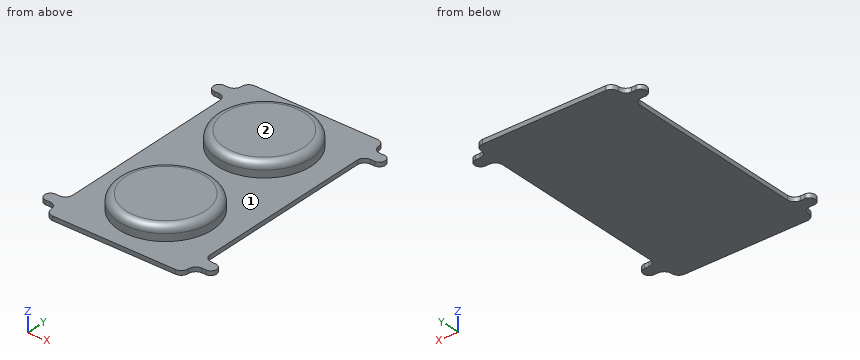
```python
from build123d import *

# Parameters (mm, degrees)
EXTRUDE_1_DEPTH = 3
FILLET_1_R      = 5
SKETCH_2_R      = 32.5
EXTRUDE_2_DEPTH = 10
FILLET_2_R      = 5


with BuildPart() as part:
    # 草圖1 → 填料-伸長1 (new body)
    with BuildSketch(Plane.XY):
        with BuildLine():
            Line((-47.5, 67), (-47.5, -67))
            Line((-47.5, -67), (-55.5, -67))
            ThreePointArc((-55.5, -67), (-59.5, -71), (-55.5, -75))
            Line((-55.5, -75), (-47.5, -75))
            Line((-47.5, -75), (-47.5, -85))
            Line((-47.5, -85), (47.5, -85))
            Line((47.5, -85), (47.5, -75))
            Line((47.5, -75), (55.5, -75))
            ThreePointArc((55.5, -75), (59.5, -71), (55.5, -67))
            Line((55.5, -67), (47.5, -67))
            Line((47.5, -67), (47.5, 67))
            Line((47.5, 67), (55.5, 67))
            ThreePointArc((55.5, 67), (59.5, 71), (55.5, 75))
            Line((55.5, 75), (47.5, 75))
            Line((47.5, 75), (47.5, 85))
            Line((47.5, 85), (-47.5, 85))
            Line((-47.5, 85), (-47.5, 75))
            Line((-47.5, 75), (-55.5, 75))
            ThreePointArc((-55.5, 75), (-59.5, 71), (-55.5, 67))
            Line((-55.5, 67), (-47.5, 67))
        make_face()
    extrude(amount=EXTRUDE_1_DEPTH)

    # 圓角1
    fillet_1_edges = [part.edges().sort_by_distance(p)[0] for p in [
        (-47.5, 85, 1.5),
        (47.5, 85, 1.5),
        (47.5, 75, 1.5),
        (47.5, 67, 1.5),
        (47.5, -67, 1.5),
        (47.5, -75, 1.5),
        (47.5, -85, 1.5),
        (-47.5, -85, 1.5),
        (-47.5, -75, 1.5),
        (-47.5, -67, 1.5),
        (-47.5, 67, 1.5),
        (-47.5, 75, 1.5),
    ]]
    fillet(fillet_1_edges, radius=FILLET_1_R - 0.0001)  # a hair under: the kernel refuses the full size

    # 草圖2 → 填料-伸長2 (add)
    with BuildSketch(Plane.XY.offset(3)):
        with Locations((0, 41.5)):
            Circle(SKETCH_2_R)
        with Locations(Location((0, -41.5, 0), (0, 0, 180))):
            Circle(SKETCH_2_R)
    extrude(amount=EXTRUDE_2_DEPTH)

    # 圓角2
    fillet_2_edges = [part.edges().sort_by_distance(p)[0] for p in [
        (-32.5, 41.5, 13),
        (32.5, -41.5, 13),
    ]]
    fillet(fillet_2_edges, radius=FILLET_2_R)


solid = part.part
```
The model under review builds one solid part; all positions refer to its coordinate system, in mm. Face numbers are marked on the shaded views. Coordinates: 2 decimals unless noted, no trailing zeros. Write each loop counter-clockwise with the first axis right and the second up, starting at its lowest first coordinate (ties: lowest second). Pieces come first, ordered by that corner, then holes.
1) The part is to be moulded in two halves that separate along Y. For the marked faces 1 and 2, say which applies: pulls with the +Y half, pulls with the -Y half, needs draft (parallel to the pull), parting line crosses it, or undercut.
2) To check wall thickness, follow probe 1 along X at (y, z) = (43, 7.25); probe 2 along Z at (x, y) = (-36.5, -24); probe 3 along Y at (x, z) = (2.5, 7.25). State the ranges of each line that lie inside material, in increasing order.
3) We need section C-C on z = 11. State the section outline as (x, y) points.
4) We need section A-A on y = -41.5. State the section outline as (x, z) points.
5) Clearance check with flat-ended pins moving along their axes: pin 1 Ø2.5 at (x, z) = (54, 1.5) entering from +Y; pin 2 Ø0.9 at (x, z) = (-53.5, 1.5) entering from -Y; pin 3 Ø1 at (x, z) = (-30, 5.5) entering from +Y. State where each tip first meets the part, or that it passes through.
6) We need section B-B on x = 0. State the section outline as (y, z) points, then the cut area to 3 significant figures.
7) We need section D-D on x = 38. State the section outline as (y, z) points.
Answer list:
1. face 1: undercut
1. face 2: needs draft
2. probe 1: x = -32.47 to 32.47
2. probe 2: z = 0 to 3
2. probe 3: y = -73.9 to -9.1, 9.1 to 73.9
3. outline: circle Ø63 at (0, -41.5); circle Ø63 at (0, 41.5)
4. outline: (-47.5, 0) - (47.5, 0) - (47.5, 3) - (32.5, 3) - (32.5, 8) arc R5 ccw to (27.5, 13) - (-27.5, 13) arc R5 ccw to (-32.5, 8) - (-32.5, 3) - (-47.5, 3) - close
5. pin 1: stops at y = 75
5. pin 2: stops at y = -75
5. pin 3: stops at y = 55.14
6. outline: (-85, 0) - (85, 0) - (85, 3) - (74, 3) - (74, 8) arc R5 ccw to (69, 13) - (14, 13) arc R5 ccw to (9, 8) - (9, 3) - (-9, 3) - (-9, 8) arc R5 ccw to (-14, 13) - (-69, 13) arc R5 ccw to (-74, 8) - (-74, 3) - (-85, 3) - close
6. area: 1,790 mm2
7. outline: (-85, 0) - (85, 0) - (85, 3) - (-85, 3) - close
